from build123d import *

# Parameters (mm, degrees)
PAD_DEPTH    = 1.5
SKETCH001_R  = 1.375
POCKET_DEPTH = 1.501
SKETCH002_W  = 17
SKETCH002_H  = 13
PAD001_DEPTH = 16
SKETCH003_W  = 21.3
SKETCH003_H  = 16
PAD002_DEPTH = 13.5
SKETCH004_W  = 81
SKETCH004_H  = 42
PAD003_DEPTH = 2
SKETCH005_W  = 55.4
SKETCH005_H  = 6
PAD004_DEPTH = 13
SKETCH006_W  = 7
SKETCH006_H  = 12.5
PAD005_DEPTH = 6
SKETCH007_R  = 3
PAD006_DEPTH = 3
SKETCH008_W  = 4
SKETCH008_H  = 22.5
PAD007_DEPTH = 5.6
SKETCH009_W  = 12
SKETCH009_H  = 4.6
PAD008_DEPTH = 12
CHAMFER_SIZE = 3
SKETCH010_R  = 2.017401
PAD009_DEPTH = 7


with BuildPart() as part:
    # Sketch → Pad (new body)
    with BuildSketch(Plane.XY):
        with BuildLine():
            Line((-39.5, 28), (39.5, 28))
            ThreePointArc((42.5, 25), (41.62132, 27.12132), (39.5, 28))
            Line((42.5, 25), (42.5, -25))
            ThreePointArc((39.5, -28), (41.62132, -27.12132), (42.5, -25))
            Line((39.5, -28), (-39.5, -28))
            ThreePointArc((-42.5, -25), (-41.62132, -27.12132), (-39.5, -28))
            Line((-42.5, -25), (-42.5, 25))
            ThreePointArc((-39.5, 28), (-41.62132, 27.12132), (-42.5, 25))
        make_face()
    extrude(amount=-PAD_DEPTH)

    # Sketch001 (on Face9 of Pad) → Pocket (cut, through all)
    with BuildSketch(Plane.XY):
        with Locations((-39, 24.5)):
            Circle(SKETCH001_R)
        with Locations((19, 24.5)):
            Circle(SKETCH001_R)
        with Locations((19, -24.5)):
            Circle(SKETCH001_R)
        with Locations((-39, -24.5)):
            Circle(SKETCH001_R)
    extrude(amount=-POCKET_DEPTH, mode=Mode.SUBTRACT)

    # Sketch002 (on Face4 of Pocket) → Pad001 (join)
    with BuildSketch(Plane.XY):
        with Locations((36, 19)):
            Rectangle(SKETCH002_W, SKETCH002_H)
        with Locations((36, 1)):
            Rectangle(SKETCH002_W, SKETCH002_H)
    extrude(amount=PAD001_DEPTH)

    # Sketch003 (on Face4 of Pad001) → Pad002 (join)
    with BuildSketch(Plane.XY):
        with Locations((33.85, -17.75)):
            Rectangle(SKETCH003_W, SKETCH003_H)
    extrude(amount=PAD002_DEPTH)

    # Sketch004 (on Face5 of Pad002) → Pad003 (join)
    with BuildSketch(Plane(origin=(0, 0, -1.5), x_dir=(1, 0, 0), z_dir=(0, 0, -1))):
        Rectangle(SKETCH004_W, SKETCH004_H)
    extrude(amount=PAD003_DEPTH)

    # Sketch005 (on Face4 of Pad003) → Pad004 (join)
    with BuildSketch(Plane.XY):
        with Locations((-10, 24.5)):
            Rectangle(SKETCH005_W, SKETCH005_H)
    extrude(amount=PAD004_DEPTH)

    # Sketch006 (on Face4 of Pad004) → Pad005 (join)
    with BuildSketch(Plane.XY):
        with Locations((11, -21.75)):
            Rectangle(SKETCH006_W, SKETCH006_H)
    extrude(amount=PAD005_DEPTH)

    # Sketch007 (on Face35 of Pad005) → Pad006 (join)
    with BuildSketch(Plane.XZ.offset(28)):
        with Locations((11, 3)):
            Circle(SKETCH007_R)
    extrude(amount=PAD006_DEPTH)

    # Sketch008 (on Face4 of Pad006) → Pad007 (join)
    with BuildSketch(Plane.XY):
        with Locations((-39.4, 0.25)):
            Rectangle(SKETCH008_W, SKETCH008_H)
    extrude(amount=PAD007_DEPTH)

    # Sketch009 (on Face50 of Pad007) → Pad008 (join)
    with BuildSketch(Plane.YZ.offset(44.5)):
        with Locations((1, 3.8)):
            Rectangle(SKETCH009_W, SKETCH009_H)
        with Locations((19, 3.8)):
            Rectangle(SKETCH009_W, SKETCH009_H)
    extrude(amount=PAD008_DEPTH)

    # Chamfer
    chamfer_edges = [part.edges().sort_by_distance(p)[0] for p in [
        (56.5, 13, 3.8),
        (14, -29.5, 3),
        (56.5, 7, 3.8),
        (56.5, -5, 3.8),
        (56.5, 25, 3.8),
    ]]
    chamfer(chamfer_edges, length=CHAMFER_SIZE)

    # Sketch010 (on Face8 of Chamfer) → Pad009 (join)
    with BuildSketch(Plane.YZ.offset(56.5)):
        with Locations((0.930018, 3.811911)):
            Circle(SKETCH010_R)
        with Locations((19.019375, 3.811911)):
            Circle(SKETCH010_R)
    extrude(amount=PAD009_DEPTH)


solid = part.part
Read the model definition and answer for the solid it produces. Units are mm, in the model's axes. A direction names the side the tool comes from. Round coordinates to 2 decimals unless told otherwise and drop trailing zeros. Order: outer loops, then holes, each group sorted by start corner. A loop starts at its lowest first (then second) coordinate and runs counter-clockwise, first axis right, second up. Notation, with made-up numbers: (11.5, 80.25) - (50.5, 80.25) arc R26 ccw to (50.5, 107.25) - close; hole circle Ø2 at (71.5, 62.5). An arc over 180 degrees is marked (long way). Use one line per item in the form item = value. Start each with the question number.
(1) The part is cut by section A-A (x = 19). Give the vertices of the cut face in (y, z) (3 decimals).
(2) Determine the mould class of faces 1 (the face through (49, 7, 4)), 2 (the face through (63.5, 1, 4)), 3 (the face through (-41.6, 27.14, -0.74)) for opening direction Y: +Y half, -Y half, draft (parallel to the pull), parting line (faces both ways), or undercut.
(3) The part is cut by section C-C (y = 9). Give the vertices of the cut face in (x, z), then the cut area to 3 significant figures.
(4) The part is cut by section D-D (x = 51.5). Give the vertices of the cut face in (y, z), then the cut area to 3 significant figures.
(5) Flat-ended cylindrical pins translate along their axes: pin 1 Ø8 at (x, z) = (37, 10) entering from -Y; pin 2 Ø6 at (y, z) = (-10, 11) entering from +X; pin 3 Ø2.5 at (x, z) = (47, 3) entering from +Y. Find the tip coordinate at first contact, or state that the pin passes through.
(6) Find the intervals of material crossed by line 1 along X through (y, z) = (24.5, -0.5) (3 decimals); line 2 along Y through (x, z) = (-39, -0.9) (3 decimals); line 3 along X through (y, z) = (-4, 0.75), in increasing order. Write a range as from..to.
(7) The part is cut by section B-B (z = 10.75). Give the vertices of the cut face in (x, y), then the cut area to 3 significant figures.
(8) For faces 4 (the face through (7.5, -22, 3)), 5 (the face through (8.79, -29.48, 5.03)), 6 (the face through (-41.4, 0, 3)), 7 (the face through (56.5, 3, 3)), 8 (the face through (36, -5.5, 8)), determine the directions among +Z, -Z, +X, -X, +Y, -Y from which every point of the face is accessible in a straight line to the end or side of a thin tool.
Checked values:
q1.outline = (-28, -1.5) - (-25.875, -1.5) - (-25.875, 0) - (-28, 0) - close; (-23.125, -1.5) - (-21, -1.5) - (-21, -3.5) - (21, -3.5) - (21, -1.5) - (23.125, -1.5) - (23.125, 0) - (-23.125, 0) - close; (25.875, -1.5) - (28, -1.5) - (28, 0) - (25.875, 0) - close
q2.face_1 = undercut
q2.face_2 = draft
q2.face_3 = +Y half
q3.outline = (-42.5, -1.5) - (-40.5, -1.5) - (-40.5, -3.5) - (40.5, -3.5) - (40.5, -1.5) - (42.5, -1.5) - (42.5, 0) - (-37.4, 0) - (-37.4, 5.6) - (-41.4, 5.6) - (-41.4, 0) - (-42.5, 0) - close
q3.area = 312 mm^2
q4.outline = (-5, 1.5) - (7, 1.5) - (7, 6.1) - (-5, 6.1) - close; (13, 1.5) - (25, 1.5) - (25, 6.1) - (13, 6.1) - close
q4.area = 110 mm^2
q5.pin_1 = -25.75
q5.pin_2 = 44.5
q5.pin_3 = 25
q6.line_1 = -42.5..-40.375, -37.625..17.625, 20.375..42.5
q6.line_2 = -28..-25.875, -23.125..23.125, 25.875..28
q6.line_3 = -41.4..-37.4, 27.5..44.5
q7.outline = (-37.7, 21.5) - (17.7, 21.5) - (17.7, 27.5) - (-37.7, 27.5) - close; (23.2, -25.75) - (44.5, -25.75) - (44.5, -9.75) - (23.2, -9.75) - close; (27.5, -5.5) - (44.5, -5.5) - (44.5, 7.5) - (27.5, 7.5) - close; (27.5, 12.5) - (44.5, 12.5) - (44.5, 25.5) - (27.5, 25.5) - close
q7.area = 1,120 mm^2
q8.face_4 = +Z, -X, -Y
q8.face_5 = -Y
q8.face_6 = +Z, -X, +Y, -Y
q8.face_7 = +X
q8.face_8 = +Z, +X
